```python
from build123d import *

# Parameters (mm, degrees)
SKETCH_1_R               = 16.4
EXTRUDE_1_DEPTH          = 23
SKETCH_2_R               = 18.3
EXTRUDE_2_DEPTH          = 21.5
SKETCH_3_R               = 6
EXTRUDE_3_DEPTH          = 6
SKETCH_4_R               = 3
EXTRUDE_4_DEPTH          = 13.8
PATTERN_CIRCULAR_1_COUNT = 6
CHAMFER_1_SIZE           = 1


with BuildPart() as part:
    # 草图1 → 凸台-拉伸1 (new body)
    with BuildSketch(Plane(origin=(0, 0, 0), x_dir=(0, 0, -1), z_dir=(1, 0, 0))):
        Circle(SKETCH_1_R)
    extrude(amount=EXTRUDE_1_DEPTH)

    # 草图2 → 凸台-拉伸2 (add)
    with BuildSketch(Plane(origin=(23, 0, 0), x_dir=(0, 0, -1), z_dir=(1, 0, 0))):
        Circle(SKETCH_2_R)
    extrude(amount=EXTRUDE_2_DEPTH)

    # 草图3 → 凸台-拉伸3 (add)
    with BuildSketch(Plane(origin=(44.5, 0, 0), x_dir=(0, 0, -1), z_dir=(1, 0, 0))):
        with Locations((7.3, 0)):
            Circle(SKETCH_3_R)
    extrude(amount=EXTRUDE_3_DEPTH)

    # 草图4 → 凸台-拉伸4 (add)
    with BuildSketch(Plane(origin=(50.5, 0, 0), x_dir=(0, 0, -1), z_dir=(1, 0, 0))):
        with Locations(Location((7.3, 0, 0), (0, 0, 180))):
            Circle(SKETCH_4_R)
    extrude(amount=EXTRUDE_4_DEPTH)

    # 草图7 → M3 螺纹孔1 (revolve, cut)
    with BuildSketch(Plane(origin=(44.5, 15.5, 0), x_dir=(0, 0, -1), z_dir=(0, 1, 0))):
        Polygon((0, 0), (0, 5.751075774), (1.25, 5), (1.25, 0), align=None)
    hole_wizard_m3_1 = revolve(axis=Axis((50.85, 15.5, 0), (-1, 0, 0)), mode=Mode.SUBTRACT)

    # 阵列(圆周)1: M3 螺纹孔1 ×6 about axis
    pattern_circular_1_axis = Axis((0, 0, 0), (1, 0, 0))
    for i in range(1, PATTERN_CIRCULAR_1_COUNT):
        add(hole_wizard_m3_1.rotate(pattern_circular_1_axis, i * 360 / PATTERN_CIRCULAR_1_COUNT), mode=Mode.SUBTRACT)

    # 倒角1
    chamfer_1_edges = [part.edges().sort_by_distance(p)[0] for p in [
        (50.5, 0, -1.3),
    ]]
    chamfer(chamfer_1_edges, length=CHAMFER_1_SIZE)


solid = part.part
```
Design review of the part built by this model. Coordinates are the model's own, in mm. A direction names the side the tool comes from. Coordinates: 2 decimals unless noted, no trailing zeros. Write each loop counter-clockwise with the first axis right and the second up, starting at its lowest first coordinate (ties: lowest second). Pieces come first, ordered by that corner, then holes. Notation, with made-up numbers: M -15.5,85.5 L 24.5,85.5 A13 ccw 24.5,105.5 Z; hole C 80,-17 d6. An arc over 180 degrees is marked long. Answer as a JSON object with one key per item and string values.
Item 1: Draft analysis for pull direction Y (two halves, no side actions). For faces 1 (the cylindrical face through (46.965, 1.802, -13.023)), 2 (the cylindrical face through (42.04, 6.64, 14)), 3 (the flat face through (0, 0, 0)), state which applies: pulls with the +Y half, pulls with the -Y half, needs draft (parallel to the pull), parting line crosses it, or undercut.
Outcome:
{"face 1": "parting line crosses it", "face 2": "undercut", "face 3": "needs draft"}
Item 2: Add section A-A, the plane y = 0. Give the boundary of the cut face in (x, z).
Outcome:
{"outline": "M 0,-16.4 L 23,-16.4 L 23,-18.3 L 44.5,-18.3 L 44.5,-13.3 L 49.5,-13.3 L 50.5,-12.3 L 50.5,-10.3 L 64.3,-10.3 L 64.3,-4.3 L 50.5,-4.3 L 50.5,-2.3 L 49.5,-1.3 L 44.5,-1.3 L 44.5,18.3 L 23,18.3 L 23,16.4 L 0,16.4 Z"}
Item 3: Wall thickness on probe 1 along Y at (x, z) = (40, 0); probe 2 along Z at (x, y) = (41, -7); probe 3 along Y at (x, z) = (45.5, -4): over which ranges is each line inside the solid? List them lowest first.
Outcome:
{"probe 1": "-18.3 to -16.75, -14.25 to 14.25, 16.75 to 18.3", "probe 2": "-16.91 to -14.42, -12.42 to 12.42, 14.42 to 16.91", "probe 3": "-5.01 to 5.01"}
Item 4: Insertion check: pin 1 Ø3 at (y, z) = (7.75, 13.42) entering from -X; pin 2 Ø1 at (x, z) = (7, -8) entering from -Y; pin 3 Ø2 at (y, z) = (15.5, 0) entering from +X; pin 4 Ø1.5 at (x, z) = (34.5, 13) entering from +Y. Each pin has a flat end and moves straight along its axis. Give the tip position at first contact, or say it passes through.
Outcome:
{"pin 1": "x = 0", "pin 2": "y = -14.58", "pin 3": "x = 39.35", "pin 4": "y = 13.6"}
Item 5: Add section B-B, the plane x = 43. Give the boundary of the cut face in (y, z).
Outcome:
{"outline": "C 0,0 d36.6; hole C -15.5,0 d2.5; hole C -7.75,-13.42 d2.5; hole C -7.75,13.42 d2.5; hole C 7.75,-13.42 d2.5; hole C 7.75,13.42 d2.5; hole C 15.5,0 d2.5"}
Item 6: Add section C-C, the plane z = -7.3. Give the boundary of the cut face in (x, y).
Outcome:
{"outline": "M 0,-14.69 L 23,-14.69 L 23,-16.78 L 44.5,-16.78 L 44.5,-6 L 49.5,-6 L 50.5,-5 L 50.5,-3 L 64.3,-3 L 64.3,3 L 50.5,3 L 50.5,5 L 49.5,6 L 44.5,6 L 44.5,16.78 L 23,16.78 L 23,14.69 L 0,14.69 Z"}
Item 7: Add section D-D, the plane x = 27. Give the boundary of the cut face in (y, z).
Outcome:
{"outline": "C 0,0 d36.6"}
Item 8: Machinability: for faces 4 (the cylindrical face through (42.035, -8.804, 12.751)), 5 (the cylindrical face through (11.34, 16.26, 2.13)), 6 (the flat face through (64.3, 0, -7)), which of the approach directions +Z, -Z, +X, -X, +Y, -Y give a long, thin tool a straight path to every point of the face, cutting with its end or side? Answer none if there is none.
Outcome:
{"face 4": "+X", "face 5": "-X", "face 6": "+Z, -Z, +X, +Y, -Y"}
